Autodesk Fusion 360 part; units mm, degrees
sketch "Sketch1" plane through (0, 0, 0) normal (1, 0, 0) x (0, 1, 0)
  line L0 (-8.75, 0) -> (-8.75, 6.9)
  line L1 (0, 0) -> (0, 67)
  line L2 (0, 0) -> (-8.75, 0)
  line L3 (-8.75, 6.9) -> (-12.35, 6.9)
  line L4 (-12.35, 6.9) -> (-12.35, 8.9)
  line L5 (-12.35, 8.9) -> (-8, 23.5)
  line L6 (-5.75, 0) -> (-5.75, 31.5)
  line L7 (-5.75, 31.5) -> (0, 31.5)
  line L8 (0, 0) -> (-13.7425, 0)
  line L9 (-8, 23.5) -> (-8, 31.5)
  line L10 (-8, 31.5) -> (-7.1919, 33.5)
  line L11 (-7.1919, 33.5) -> (0, 33.5)
  dimension "d1" = 8.75
  dimension "d2" = 13.7425
  dimension "d3" = 6.9
  dimension "d4" = 3.6
  dimension "d5" = 2
  dimension "d6" = 3
  dimension "d8" = 31.5
  dimension "d10" = 8
  dimension "d11" = 8
  dimension "d13" = 8
  dimension "d25" = 22
  dimension "d26" = 2
  dimension "d27" = 2
revolve "Revolve1" add sketch "Sketch1" angle 360 about axis through (0, 0, 0) along (0, 0, 1) contours L0 L1 L2 L3 L4 L5 L6 L7 L8 L9 L10 L11
sketch "Sketch2" plane through (0, 0, 0) normal (1, 0, 0) x (0, 1, 0)
  line L0 (-8.75, 3) -> (-10.25, 3)
  line L1 (-10.25, 3) -> (-10.25, 0)
  line L2 (-10.25, 0) -> (-8.75, 0)
  line L3 (-8.75, 0) -> (-8.75, 3)
  line L4 (-8.75, 0) -> (-8.75, 6.9)
  line L5 (-8.75, 3) -> (-7.5, 3)
  line L6 (-7.5, 3) -> (-7.5, 0)
  line L7 (-7.5, 0) -> (-8.75, 0)
  line L8 (-8.75, 0) -> (-8.75, 3)
  dimension "d15" = 3
  dimension "d16" = 1.5
extrude "Extrude1" add sketch "Sketch2" along normal mid plane 3.5
mirror "Mirror1" about plane through (0, 0, 0) normal (0, 1, 0) of "Revolve1", "Extrude1"
fillet "Fillet1" radius 0.5 6 edges at (-1.75, -10.25, 1.5) (0, -10.25, 3) (1.75, -10.25, 1.5) (1.75, 10.25, 1.5) (0, 10.25, 3) (-1.75, 10.25, 1.5)
chamfer "Chamfer1" distance 1 angle 30 1 edges at (-5.3609, -2.0793, 31.5) measured on face at (-0.5725, -5.7214, 21)
equation "d1 = ( 17.5 / 2 ) * 1 mm"
equation "d17 = ( 3.5 / 2 ) * 1 mm"
Can you work these out from the model? Positions are in its coordinate system, mm. A direction names the side the tool comes from. Round coordinates to 2 decimals unless told otherwise and drop trailing zeros. Loops run counter-clockwise (first coordinate to the right, second up) from the corner with the lowest first, then second, coordinate; pieces in that order, holes last. Notation, with made-up numbers: (55.5, 53) - (98.5, 53) arc R19 cw to (98.5, 82) - close; hole circle Ø5 at (17.5, 55.5). An arc over 180 degrees is marked (long way). Answer in a Markdown table with one row per item. Add a question column.
Q1. I want a section at D-D on z = 17.5. List the corners of the cut face in (x, y) for me.
Q2. I want a section at B-B on x = 0. List the corners of the cut face in (y, z) for me, and give its area (3 significant figures).
Q3. We'd pull the mould along Z, two halves only. Please class faces 1 (the flat face through (0, -9, 3)), 2 (the flat face through (-1.75, -9, 2)), 3 (the flat face through (0, 9, 3)), 4 (the flat face through (0, 0, 31.5)): pulls with the +Z half, pulls with the -Z half, needs draft (parallel to the pull), parting line crosses it, or undercut.
Q4. I want a section at A-A on y = 0. List the corners of the cut face in (x, z) for me.
Q5. For pin 1 Ø4 at (x, z) = (-6.5, 5.5) entering from -Y; pin 2 Ø3 at (y, z) = (3, 27) entering from +X; pin 3 Ø12 at (x, z) = (2, 23.5) entering from +Y, each with a flat end and sliding along its axis, tell me the tip position at first contact or that it passes through.
Q6. I want a section at C-C on z = 26. List the corners of the cut face in (x, y) for me, and give its area (3 significant figures).
Q7. I need wall thicknesses on L1, parallel to Z at x = -2, y = 4.75; L2, parallel to X at y = 0, z = 21.5; L3, parallel to Y at x = 3.75, z = 21. Which ranges of each line are inside material? Lowest first, please.
Q8. Which directions (+Z, -Z, +X, -X, +Y, -Y) give clear straight access to the entire face, cutting with the end or side of a thin tool? Please do faces 5 (the cylindrical face through (-7.81, 1.73, 27.56)), 6 (the flat face through (0, -10.25, 1)), 7 (the cylindrical face through (5.7, 0.75, 15.46)), 8 (the flat face through (1.75, 9, 2)).
A:
| question | item | result |
|---|---|---|
| 1 | outline | circle Ø19.58 at (0, 0); hole circle Ø11.5 at (0, 0) |
| 2 | outline | (-12.35, 6.9) - (-8.75, 6.9) - (-8.75, 3) - (-9.75, 3) arc R0.5 ccw to (-10.25, 2.5) - (-10.25, 0) - (-5.75, 0) - (-5.75, 30.5) - (-5.17, 31.5) - (5.17, 31.5) - (5.75, 30.5) - (5.75, 0) - (10.25, 0) - (10.25, 2.5) arc R0.5 ccw to (9.75, 3) - (8.75, 3) - (8.75, 6.9) - (12.35, 6.9) - (12.35, 8.9) - (8, 23.5) - (8, 31.5) - (7.19, 33.5) - (-7.19, 33.5) - (-8, 31.5) - (-8, 23.5) - (-12.35, 8.9) - close |
| 2 | area | 273 mm^2 |
| 3 | face 1 | undercut |
| 3 | face 2 | needs draft |
| 3 | face 3 | undercut |
| 3 | face 4 | pulls with the -Z half |
| 4 | outline | (-12.35, 6.9) - (-8.75, 6.9) - (-8.75, 0) - (-5.75, 0) - (-5.75, 30.5) - (-5.17, 31.5) - (5.17, 31.5) - (5.75, 30.5) - (5.75, 0) - (8.75, 0) - (8.75, 6.9) - (12.35, 6.9) - (12.35, 8.9) - (8, 23.5) - (8, 31.5) - (7.19, 33.5) - (-7.19, 33.5) - (-8, 31.5) - (-8, 23.5) - (-12.35, 8.9) - close |
| 5 | pin 1 | y = -11.26 |
| 5 | pin 2 | x = 7.86 |
| 5 | pin 3 | y = 9.72 |
| 6 | outline | circle Ø16 at (0, 0); hole circle Ø11.5 at (0, 0) |
| 6 | area | 97.2 mm^2 |
| 7 | L1 | 31.5 to 33.5 |
| 7 | L2 | -8.6 to -5.75, 5.75 to 8.6 |
| 7 | L3 | -7.9 to -4.36, 4.36 to 7.9 |
| 8 | face 5 | +Z |
| 8 | face 6 | -Z, +X, -X, -Y |
| 8 | face 7 | -Z |
| 8 | face 8 | -Z, +X, +Y |
